```python
from build123d import *
from build123d.topology import SkipClean

# Parameters (mm, degrees)
SKETCH_1_W          = 15.717143143
SKETCH_1_H          = 6
CUT_EXTRUDE_START   = -11.070751878
CUT_EXTRUDE_1_DEPTH = 22.141503755
SKETCH_4_R          = 4
CUT_EXTRUDE_2_DEPTH = 21
SKETCH_6_R          = 4
CUT_EXTRUDE_3_DEPTH = 21


# Read off the part's stored shape, not the designer's step: the extrude step
with BuildPart() as part:
    # Sketch 1 → Revolve 3 (revolve)
    with SkipClean():  # the faces are left unmerged after this step: merging them gives an invalid solid
        with BuildSketch(Plane.XY, mode=Mode.PRIVATE) as revolve_3_sk:
            with BuildLine():
                ThreePointArc((8.569714114, -8.4), (11.109378231, -4.536707541), (12, 0))
                Line((12, 0), (4, 0))
                ThreePointArc((4, 0), (0, -4), (-4, 0))
                Line((-4, 0), (-12, 0))
                ThreePointArc((-12, 0), (-4.536707541, -11.109378231), (8.569714114, -8.4))
            make_face()
            with BuildLine():
                Line((4, 0), (12, 0))
                ThreePointArc((12, 0), (11.109378231, 4.536707541), (8.569714114, 8.4))
                ThreePointArc((8.569714114, 8.4), (-4.536707541, 11.109378231), (-12, 0))
                Line((-12, 0), (-4, 0))
                ThreePointArc((-4, 0), (0, 4), (4, 0))
            make_face()
            with BuildLine():
                Line((12, 0), (14.282856857, 0))
                Line((14.282856857, 0), (14.282856857, 6))
                ThreePointArc((14.282856857, 6), (11.18447018, 6.624364434), (8.569714114, 8.4))
                ThreePointArc((8.569714114, 8.4), (11.109378231, 4.536707541), (12, 0))
            make_face()
            with Locations((22.141428429, 3)):
                Rectangle(SKETCH_1_W, SKETCH_1_H)
            Polygon((30, 0), (36, 0), (36, 4), (36, 8.5), (30, 8.5), (30, 6), align=None)
        revolve(revolve_3_sk.sketch.rotate(Axis((36, 0, 0), (-1, 0, 0)), 270), axis=Axis((36, 0, 0), (-1, 0, 0)))

    # Cut-Extrude 1 outline → Cut-Extrude 1 (cut)
    with SkipClean():  # the faces are left unmerged after this step: merging them gives an invalid solid
        with BuildSketch(Plane(origin=(0, 0, 0), x_dir=(1, 0, 0), z_dir=(0, 1, 0)).offset(CUT_EXTRUDE_START)):
            with BuildLine():
                Line((12.79642365, 4.513566798), (14.282856857, 6))
                Line((14.282856857, 6), (5.630326424, 10.597142276))
                ThreePointArc((5.630326424, 10.597142276), (-3.985808775, 11.318715851), (-11.028032544, 4.73101451))
                Line((-11.028032544, 4.73101451), (-6.481391111, 4.68951696))
                Line((-6.481391111, 4.68951696), (12.79642365, 4.513566798))
            make_face()
            with BuildLine():
                Line((5.630326419, -10.597142274), (14.282856857, -6))
                Line((14.282856857, -6), (12.796423652, -4.513566795))
                Line((12.796423652, -4.513566795), (-6.481391109, -4.689516958))
                Line((-6.481391109, -4.689516958), (-11.028032543, -4.731014508))
                ThreePointArc((-11.028032543, -4.731014508), (-3.985808776, -11.318715845), (5.630326419, -10.597142274))
            make_face()
        extrude(amount=CUT_EXTRUDE_1_DEPTH, mode=Mode.SUBTRACT)

    # Sketch 3 → Revolve 6 (revolve)
    with SkipClean():  # the faces are left unmerged after this step: merging them gives an invalid solid
        with BuildSketch(Plane(origin=(0, 0, 0), x_dir=(1, 0, 0), z_dir=(0, 1, 0))):
            with BuildLine():
                Line((0, 4.623306587), (6.570843405, 4.563333972))
                ThreePointArc((6.570843405, 4.563333972), (5.974513841, 5.320261682), (5.291502622, 6))
                Line((5.291502622, 6), (0, 6))
                Line((0, 6), (0, 4.623306587))
            make_face()
            Polygon((6.570843405, -4.563333972), (6.570843405, 4.563333972), (0, 4.623306587), (0, -4.623306587), align=None)
            with BuildLine():
                ThreePointArc((5.291502622, -6), (5.974513841, -5.320261682), (6.570843405, -4.563333972))
                Line((6.570843405, -4.563333972), (0, -4.623306587))
                Line((0, -4.623306587), (0, -6))
                Line((0, -6), (5.291502622, -6))
            make_face()
        revolve(axis=Axis((0, 0, -6), (0, 0, 1)))

    # Sketch 4 → Cut-Extrude 2 (cut)
    with SkipClean():  # the faces are left unmerged after this step: merging them gives an invalid solid
        with BuildSketch(Plane(origin=(0, 0, -6), x_dir=(-1, 0, 0), z_dir=(0, 0, -1))):
            Circle(SKETCH_4_R)
        extrude(amount=-CUT_EXTRUDE_2_DEPTH, mode=Mode.SUBTRACT)

    # Sketch 6 → Cut-Extrude 3 (cut)
    with SkipClean():  # the faces are left unmerged after this step: merging them gives an invalid solid
        with BuildSketch(Plane(origin=(36, 0, 0), x_dir=(0, 0, -1), z_dir=(1, 0, 0))):
            Circle(SKETCH_6_R)
        extrude(amount=-CUT_EXTRUDE_3_DEPTH, mode=Mode.SUBTRACT)


solid = part.part
```
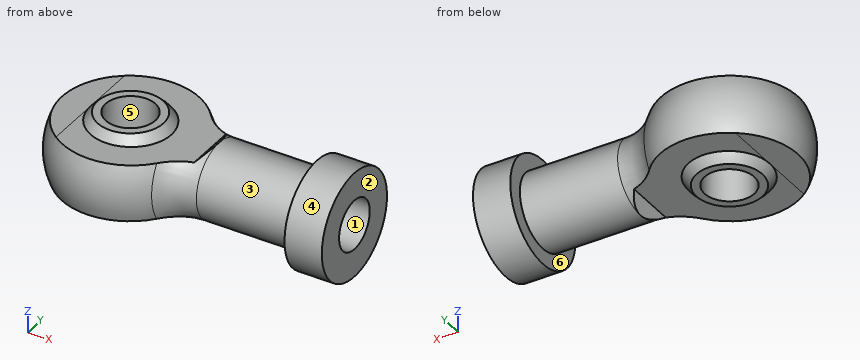
For this review, take the finished solid that the model builds, in its own axes (mm). Face numbers are marked on the shaded views. A direction names the side the tool comes from. Round coordinates to 2 decimals unless told otherwise and drop trailing zeros. Loops run counter-clockwise (first coordinate to the right, second up) from the corner with the lowest first, then second, coordinate; pieces in that order, holes last.
Q1. Add section C-C on x = 30.5. Write out the cut boundary in (y, z).
Result sheet:
outline: circle Ø17 at (0, 0); hole circle Ø8 at (0, 0)
Q2. Mouldability with a two-part tool opening along Y and no side actions: class the marked faces 4, 5 and 6 as +Y half, -Y half, draft (parallel to the pull), parting line (faces both ways), or undercut.
Result sheet:
face 4: parting line
face 5: undercut
face 6: draft
Q3. To check wall thickness, follow line 1 along Y through (x, z) = (27, 0); line 2 along Y through (x, z) = (31, 0); line 3 along Z through (x, y) = (24.5, -0.25). State the ranges of each line that lie inside material, in increasing order.
Result sheet:
line 1: y = -6 to -4, 4 to 6
line 2: y = -8.5 to -4, 4 to 8.5
line 3: z = -5.99 to -3.99, 3.99 to 5.99
Q4. Machinability: for the marked faces 1, 2 and 3, which of the approach directions +Z, -Z, +X, -X, +Y, -Y give a long, thin tool a straight path to every point of the face, cutting with its end or side? Answer none if there is none.
Result sheet:
face 1: +X
face 2: +Z, -Z, +X, +Y, -Y
face 3: none
Q5. Add section D-D on z = 5.25. Give the number of separate pieces and of enclosed holes in the cut face, plus the area to 3 significant figures.
Result sheet:
separate pieces: 2
enclosed holes: 1
area: 240 mm2
Q6. Add section A-A on z = 0. Write out the cut boundary in (x, y).
Result sheet:
outline: (8.57, -8.4) arc R8 cw to (14.28, -6) - (30, -6) - (30, -8.5) - (36, -8.5) - (36, -4) - (15, -4) - (15, 4) - (36, 4) - (36, 8.5) - (30, 8.5) - (30, 6) - (14.28, 6) arc R8 cw to (8.57, 8.4) arc R12 ccw (long way) to start; hole circle Ø8 at (0, 0)
Q7. Insertion check: pin 1 Ø10 at (x, z) = (-4.5, -6.5) entering from -Y; pin 2 Ø10.5 at (x, y) = (0, 0) entering from -Z; pin 3 Ø9 at (y, z) = (0.5, -1.5) entering from +X; pin 4 Ø6 at (x, y) = (16, -5) entering from +Z. Each pin has a flat end and moves straight along its axis. Give the tip position at first contact, or say it passes through.
Result sheet:
pin 1: stops at y = -11.64
pin 2: stops at z = -6
pin 3: stops at x = 36
pin 4: stops at z = 5.66
Q8. Add section B-B on x = -0.5. Write out the cut boundary in (y, z), plus the area to 3 significant figures.
Result sheet:
outline: (-11.06, -4.63) - (-6.5, -4.63) arc R7.98 ccw to (-5.27, -6) - (-3.97, -6) - (-3.97, 6) - (-5.27, 6) arc R7.98 ccw to (-6.5, 4.63) - (-11.06, 4.63) arc R11.99 ccw to start; (3.97, -6) - (5.27, -6) arc R7.98 ccw to (6.5, -4.63) - (11.06, -4.63) arc R11.99 ccw to (11.06, 4.63) - (6.5, 4.63) arc R7.98 ccw to (5.27, 6) - (3.97, 6) - close
area: 154 mm2
